from build123d import *

# Parameters (mm, degrees)
SKETCH1_R                   = 6.35
BOSS_EXTRUDE1_DEPTH         = 200.025
F_1_4_28_TAPPED_HOLE6_D     = 5.4102
F_1_4_28_TAPPED_HOLE6_DEPTH = 29.972
F_1_4_28_TAPPED_HOLE6_TIP   = 1.625388061
F_1_4_28_TAPPED_HOLE8_D     = 5.4102
F_1_4_28_TAPPED_HOLE8_DEPTH = 29.972
F_1_4_28_TAPPED_HOLE8_TIP   = 1.625388061
FILLET4_R                   = 2.54
FILLET5_R                   = 2.54


with BuildPart() as part:
    # Sketch1 → Boss-Extrude1 (new body)
    with BuildSketch(Plane(origin=(0, 0, 0), x_dir=(1, 0, 0), z_dir=(0, 1, 0))):
        with Locations(Location((0, 0, 0), (0, 0, 90))):
            Circle(SKETCH1_R)
    extrude(amount=BOSS_EXTRUDE1_DEPTH)

    # 1/4-28 Tapped Hole6
    with Locations(Plane.ZX.offset(200.025)):
        with Locations((0, 0)):
            Hole(F_1_4_28_TAPPED_HOLE6_D / 2, depth=F_1_4_28_TAPPED_HOLE6_DEPTH)
            with Locations((0, 0, -(F_1_4_28_TAPPED_HOLE6_DEPTH + F_1_4_28_TAPPED_HOLE6_TIP / 2))):  # 118° drill point
                Cone(0, F_1_4_28_TAPPED_HOLE6_D / 2, F_1_4_28_TAPPED_HOLE6_TIP, mode=Mode.SUBTRACT)

    # 1/4-28 Tapped Hole8
    with Locations(Plane(origin=(0, 0, 0), x_dir=(0, 0, -1), z_dir=(0, -1, 0))):
        with Locations((0, 0)):
            Hole(F_1_4_28_TAPPED_HOLE8_D / 2, depth=F_1_4_28_TAPPED_HOLE8_DEPTH)
            with Locations((0, 0, -(F_1_4_28_TAPPED_HOLE8_DEPTH + F_1_4_28_TAPPED_HOLE8_TIP / 2))):  # 118° drill point
                Cone(0, F_1_4_28_TAPPED_HOLE8_D / 2, F_1_4_28_TAPPED_HOLE8_TIP, mode=Mode.SUBTRACT)

    # Fillet4
    fillet4_edges = [part.edges().sort_by_distance(p)[0] for p in [
        (0, 200.025, 6.35),
    ]]
    fillet(fillet4_edges, radius=FILLET4_R)

    # Fillet5
    fillet5_edges = [part.edges().sort_by_distance(p)[0] for p in [
        (0, 0, 6.35),
    ]]
    fillet(fillet5_edges, radius=FILLET5_R)


solid = part.part
Verification items for the finished model (mm, model axes). A direction names the side the tool comes from. Coordinates: 2 decimals unless noted, no trailing zeros. Order: outer loops, then holes, each group sorted by start corner. A loop starts at its lowest first (then second) coordinate and runs counter-clockwise, first axis right, second up. Notation, with made-up numbers: M 6.25,37 L 17.25,37 A13 ccw 17.25,43 Z; hole C 54,33.5 d8. An arc over 180 degrees is marked long. Write each question's results on one line, items separated by ' | '.
1) Section check A-A on y = 20.5. Record the cut outline in (x, z), plus the area to 3 significant figures.
Solved:
outline: C 0,0 d12.7; hole C 0,0 d5.41 | area: 104 mm²
2) Release check for a two-part mould opening along X. For faces 1 (the face through (1, 200.025, 3)), 2 (the face through (-0.459, 31.315, 0.102)), 3 (the face through (0.81, 15.2, 2.58)), 4 (the face through (3.86, 98.65, 5.04)) record: pulls with the +X half, pulls with the -X half, needs draft (parallel to the pull), parting line crosses it, or undercut.
Solved:
face 1: needs draft | face 2: undercut | face 3: undercut | face 4: parting line crosses it
3) Section check B-B on y = 77. Record the cut outline in (x, z), plus the area to 3 significant figures.
Solved:
outline: C 0,0 d12.7 | area: 127 mm²
4) Gauge pin test, flat ends, axial feed: pin 1 Ø3 at (y, z) = (159.5, 4) entering from -X; pin 2 Ø3 at (x, y) = (4.5, 48) entering from +Z; pin 3 Ø1 at (y, z) = (161.5, 2) entering from +X. Record the tip position at first contact, or that the pin passes through.
Solved:
pin 1: stops at x = -5.84 | pin 2: stops at z = 5.6 | pin 3: stops at x = 6.17
5) Scan lines: line 1 along X through (y, z) = (181, 0); line 2 along Z through (x, y) = (-1, 24); line 3 along Y through (x, z) = (-1.75, -3.75). Record each from-to range of solid material in increasing order. Write a range as [from, to].
Solved:
line 1: x = [-6.35, -2.71], [2.71, 6.35] | line 2: z = [-6.27, -2.51], [2.51, 6.27] | line 3: y = [0.02, 200]
6) Access from +Z, -Z, +X, -X, +Y, -Y to the whole of each face (thin tool, end or side, straight path). Record for faces 5 (the face through (1, 0, 3)), 6 (the face through (0.81, 184.83, -2.58)).
Solved:
face 5: +Z, -Z, +X, -X, -Y | face 6: +Y
